```python
from build123d import *

# Parameters (mm, degrees)
VYSUNOUT1_DEPTH          = 6
ODEBRAT_START            = -29.5
ODEBRAT_VYSUNUT_M2_DEPTH = 3.5


# Read off the part's stored shape, not the designer's step: Odebrat vysunutím2
with BuildPart() as part:
    # Skica1 → Vysunout1 (new, symmetric)
    with BuildSketch(Plane.XY):
        Polygon((-8.5, 0), (21, 0), (21, 20), (26.5, 20), (26.5, 22), (21, 22), (21, 26), (-8.5, 26), (-8.5, 22), (-14, 22), (-14, 20), (-8.5, 20), align=None)
    extrude(amount=VYSUNOUT1_DEPTH, both=True)

    # Skica2 → Rotovat1 (revolve)
    with BuildSketch(Plane.XY, mode=Mode.PRIVATE) as rotovat1_sk:
        Polygon((-6.5, 26), (-6.5, 29.5), (-4, 29.5), (-4, 32.4), (-8.5, 32.4), (-8.5, 34), (-3.5, 34), (-3.5, 35), (0, 35), (0, 26), align=None)
    revolve(rotovat1_sk.sketch.rotate(Axis((0, 0, 0), (0, 1, 0)), 270), axis=Axis((0, 0, 0), (0, 1, 0)))

    # Odebrat vysunutím2 outline → Odebrat vysunutím2 (cut)
    with BuildSketch(Plane.XZ.offset(ODEBRAT_START)):
        with BuildLine():
            Line((-2.5, 6), (2.5, 6))
            ThreePointArc((2.5, 6), (0, 6.5), (-2.5, 6))
        make_face()
        with BuildLine():
            Line((2.5, -6), (-2.5, -6))
            ThreePointArc((-2.5, -6), (0, -6.5), (2.5, -6))
        make_face()
    extrude(amount=ODEBRAT_VYSUNUT_M2_DEPTH, mode=Mode.SUBTRACT)


solid = part.part
```
The model under review builds one solid part; all positions refer to its coordinate system, in mm. A direction names the side the tool comes from. Round coordinates to 2 decimals unless told otherwise and drop trailing zeros. Loops run counter-clockwise (first coordinate to the right, second up) from the corner with the lowest first, then second, coordinate; pieces in that order, holes last. Notation, with made-up numbers: (45.25, 12.5) - (81.25, 12.5) arc R15 cw to (81.25, 19.5) - close; hole circle Ø8 at (-19.75, -40). An arc over 180 degrees is marked (long way). Use a Markdown table: item, result. Add a question column.
Q1. Machinability: for faces 1 (the face through (2, 32.4, 4)), 2 (the face through (21, 24, 0)), 3 (the face through (21, 10, 0)), which of the approach directions +Z, -Z, +X, -X, +Y, -Y give a long, thin tool a straight path to every point of the face, cutting with its end or side? Answer none if there is none.
Q2. Add section C-C (z = -2.75). State the section outline as (x, y) points.
Q3. Insertion check: pin 1 Ø10 at (x, y) = (-6, 16.5) entering from -Z; pin 2 Ø1.6 at (x, z) = (-12, 0) entering from -Y; pin 3 Ø6.5 at (x, z) = (-5, -2.5) entering from +Y; pin 4 Ø9.5 at (y, z) = (11.5, -1) entering from -X. Each pin has a flat end and moves straight along its axis. Give the tip position at first contact, or say it passes through.
Q4. The part is to be moulded in two halves that separate along Y. For faces 4 (the face through (-8.5, 10, 0)), 5 (the face through (-3, 29.5, 3)), 6 (the face through (6, 0, 0)), say which applies: pulls with the +Y half, pulls with the -Y half, needs draft (parallel to the pull), parting line crosses it, or undercut.
Q5. Add section B-B (x = 0). State the section outline as (y, z) points.
Q6. Add section A-A (x = -5). State the section outline as (y, z) points.
Q7. For probe 1 along Y at (x, z) = (-4, 1.5); probe 2 along X at (y, z) = (8.5, -1.5); probe 3 along Z at (x, y) = (12, 2), list the stretches that pass through material, from the lowest coordinate up.
Q8. Add section D-D (y = 27). State the section outline as (x, z) points, plus the area to 3 significant figures.
Worked answers:
| question | item | result |
|---|---|---|
| 1 | face 1 | none |
| 1 | face 2 | +Z, -Z, +X, +Y |
| 1 | face 3 | +Z, -Z, +X, -Y |
| 2 | outline | (-14, 20) - (-8.5, 20) - (-8.5, 0) - (21, 0) - (21, 20) - (26.5, 20) - (26.5, 22) - (21, 22) - (21, 26) - (5.89, 26) - (5.89, 29.5) - (2.9, 29.5) - (2.9, 32.4) - (8.04, 32.4) - (8.04, 34) - (2.17, 34) - (2.17, 35) - (-2.17, 35) - (-2.17, 34) - (-8.04, 34) - (-8.04, 32.4) - (-2.9, 32.4) - (-2.9, 29.5) - (-5.89, 29.5) - (-5.89, 26) - (-8.5, 26) - (-8.5, 22) - (-14, 22) - close |
| 3 | pin 1 | z = -6 |
| 3 | pin 2 | y = 20 |
| 3 | pin 3 | y = 35 |
| 3 | pin 4 | x = -8.5 |
| 4 | face 4 | needs draft |
| 4 | face 5 | undercut |
| 4 | face 6 | pulls with the -Y half |
| 5 | outline | (0, -6) - (29.5, -6) - (29.5, -4) - (32.4, -4) - (32.4, -8.5) - (34, -8.5) - (34, -3.5) - (35, -3.5) - (35, 3.5) - (34, 3.5) - (34, 8.5) - (32.4, 8.5) - (32.4, 4) - (29.5, 4) - (29.5, 6) - (0, 6) - close |
| 6 | outline | (0, -6) - (26, -6) - (26, -4.15) - (29.5, -4.15) - (29.5, 4.15) - (26, 4.15) - (26, 6) - (0, 6) - close; (32.4, -6.87) - (34, -6.87) - (34, 6.87) - (32.4, 6.87) - close |
| 7 | probe 1 | 0 to 29.5, 32.4 to 34 |
| 7 | probe 2 | -8.5 to 21 |
| 7 | probe 3 | -6 to 6 |
| 8 | outline | (-2.5, -6) - (2.5, -6) arc R6.5 ccw to (2.5, 6) - (-2.5, 6) arc R6.5 ccw to start |
| 8 | area | 129 mm² |
